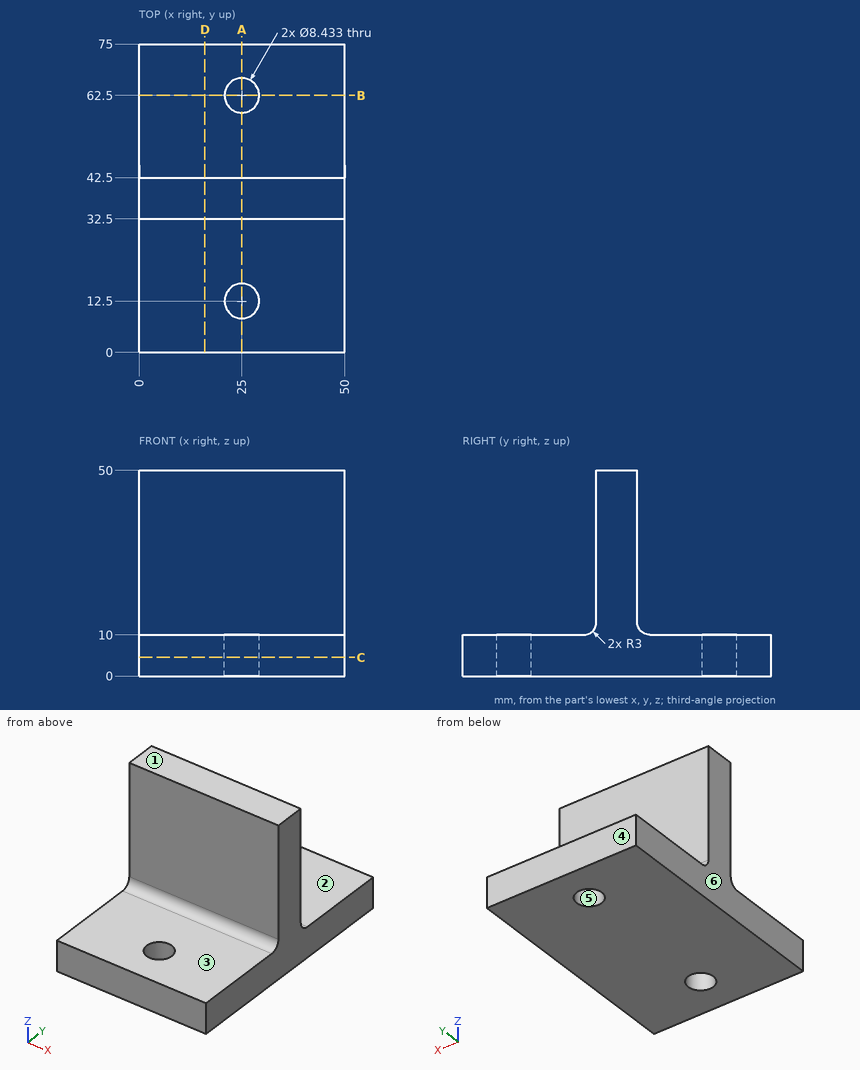
Can you work these out from the drawing? Everything is in mm from the part's minimum corner. A direction names the side the tool comes from. Coordinates: 2 decimals unless noted, no trailing zeros. Loops run counter-clockwise (first coordinate to the right, second up) from the corner with the lowest first, then second, coordinate; pieces in that order, holes last. Notation, with made-up numbers: M 87.25,5 L 125.25,5 A31 cw 125.25,29 Z; hole C 43,-1.5 d11. An arc over 180 degrees is marked long. One line per item, written item: value.
1. Will these pins go through, and if not, where does the flat tip stop? pin 1 Ø10 at (x, z) = (20, 27.5) entering from -Y; pin 2 Ø3 at (x, y) = (44, 15.5) entering from +Z; pin 3 Ø5 at (x, y) = (25, 62.5) entering from -Z.
Geometry says:
pin 1: stops at y = 32.5
pin 2: stops at z = 10
pin 3: passes through
2. Imagine slicing it at C-C (z = 4.5). List the corners of the cut face in (x, y) for me, and give its area (3 significant figures).
Geometry says:
outline: M 0,0 L 50,0 L 50,75 L 0,75 Z; hole C 25,12.5 d8.43; hole C 25,62.5 d8.43
area: 3,640 mm2
3. Imagine slicing it at D-D (x = 16). List the corners of the cut face in (y, z) for me, and give its area (3 significant figures).
Geometry says:
outline: M 0,0 L 75,0 L 75,10 L 45.5,10 A3 cw 42.5,13 L 42.5,50 L 32.5,50 L 32.5,13 A3 cw 29.5,10 L 0,10 Z
area: 1,150 mm2
4. Imagine slicing it at B-B (y = 62.5). List the corners of the cut face in (x, z) for me, and give its area (3 significant figures).
Geometry says:
outline: M 0,0 L 20.78,0 L 20.78,10 L 0,10 Z; M 29.22,0 L 50,0 L 50,10 L 29.22,10 Z
area: 416 mm2
5. On a 3-axis mill with a long thin cutter (end or side, diameter ignored), from which of +Z, -Z, +X, -X, +Y, -Y can I reach the whole of each face in a straight line? I mean the marked faces 1, 2 and 3. Say none if no direction works.
Geometry says:
face 1: +Z, +X, -X, +Y, -Y
face 2: +Z, +X, -X, +Y
face 3: +Z, +X, -X, -Y
6. Thinking about a two-plate mould opening in X: for the marked faces 4, 5 and 6, which applies, +X half, -X half, draft (parallel to the pull), parting line (faces both ways), or undercut?
Geometry says:
face 4: draft
face 5: undercut
face 6: -X half
7. Please list where these lines run through material, in increasing order: probe 1 along Y at (x, z) = (25, 4); probe 2 along Y at (x, z) = (28.5, 4.5); probe 3 along Z at (x, y) = (32.5, 10).
Geometry says:
probe 1: y = 0 to 8.28, 16.72 to 58.28, 66.72 to 75
probe 2: y = 0 to 10.15, 14.85 to 60.15, 64.85 to 75
probe 3: z = 0 to 10
8. Imagine slicing it at A-A (x = 25). List the corners of the cut face in (y, z) for me.
Geometry says:
outline: M 0,0 L 8.28,0 L 8.28,10 L 0,10 Z; M 16.72,0 L 58.28,0 L 58.28,10 L 45.5,10 A3 cw 42.5,13 L 42.5,50 L 32.5,50 L 32.5,13 A3 cw 29.5,10 L 16.72,10 Z; M 66.72,0 L 75,0 L 75,10 L 66.72,10 Z
